Here's how the part is built. I have some questions about the finished solid (model axes, mm). Round coordinates to 2 decimals unless told otherwise and drop trailing zeros. Loops run counter-clockwise (first coordinate to the right, second up) from the corner with the lowest first, then second, coordinate; pieces in that order, holes last. Notation, with made-up numbers: M 67,-38.75 L 103,-38.75 A20 ccw 103,-31.75 Z; hole C 16,7.25 d9. An arc over 180 degrees is marked long. Use a Markdown table: item, result.
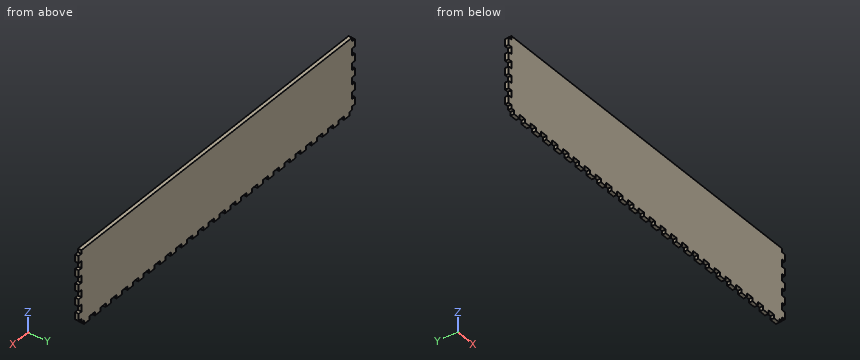
```python
from build123d import *

# Parameters (mm, degrees)
SKETCH001_W             = 500
SKETCH001_H             = 100
PAD001_DEPTH            = 5
SKETCH022_W             = 10
SKETCH022_H             = 5
PAD020_DEPTH            = 5
LINEARPATTERN002_COUNT  = 25
LINEARPATTERN002_PITCH  = 20
SKETCH023_W             = 10
SKETCH023_H             = 5
PAD021_DEPTH            = 5
LINEARPATTERN003_COUNT  = 5
LINEARPATTERN003_PITCH  = 20
SKETCH024_W             = 10
SKETCH024_H             = 5
PAD022_DEPTH            = 5
LINEARPATTERN004_COUNT  = 5
LINEARPATTERN004_PITCH  = 20
BODY001_PLACEMENT_ANGLE = 90


with BuildPart() as part:
    # Sketch001 → Pad001 (new body)
    with BuildSketch(Plane.XY):
        Rectangle(SKETCH001_W, SKETCH001_H)
    extrude(amount=PAD001_DEPTH)

    # Sketch022 (on DatumPlane) → Pad020 (join)
    with BuildSketch(Plane.XZ.offset(50)):
        with Locations((-240, 2.5)):
            Rectangle(SKETCH022_W, SKETCH022_H)
    pad020 = extrude(amount=PAD020_DEPTH)

    # LinearPattern002: Pad020 ×25
    with Locations(*[(i * LINEARPATTERN002_PITCH, 0, 0) for i in range(1, LINEARPATTERN002_COUNT)]):
        add(pad020)

    # Sketch023 (on DatumPlane) → Pad021 (join)
    with BuildSketch(Plane.YZ.offset(250)):
        with Locations((-40, 2.5)):
            Rectangle(SKETCH023_W, SKETCH023_H)
    pad021 = extrude(amount=PAD021_DEPTH)

    # LinearPattern003: Pad021 ×5
    with Locations(*[(0, i * LINEARPATTERN003_PITCH, 0) for i in range(1, LINEARPATTERN003_COUNT)]):
        add(pad021)

    # Sketch024 (on DatumPlane) → Pad022 (join)
    with BuildSketch(Plane(origin=(-250, 0, 0), x_dir=(0, -1, 0), z_dir=(-1, 0, 0))):
        with Locations((-40, 2.5)):
            Rectangle(SKETCH024_W, SKETCH024_H)
    pad022 = extrude(amount=PAD022_DEPTH)

    # LinearPattern004: Pad022 ×5
    with Locations(*[(0, -i * LINEARPATTERN004_PITCH, 0) for i in range(1, LINEARPATTERN004_COUNT)]):
        add(pad022)


with BuildPart() as part_1:
    # Body001 placement: moved
    add(part.part.moved(Location((0, 150, 55))).rotate(Axis((0, 150, 55), (1, 0, 0)), BODY001_PLACEMENT_ANGLE))


solid = part_1.part
```
Q1. Will these pins go through, and if not, where does the flat tip stop? P1, Ø2.5, axis at x = 210.5, y = 148, coming from the -Z side; P2, Ø2.5, axis at y = 146.5, z = 3.5, coming from the -X side; P3, Ø2.5, axis at y = 147.5, z = 7.5, coming from the -X side.
Return value:
| item | result |
|---|---|
| P1 | stops at z = 5 |
| P2 | stops at x = -245 |
| P3 | stops at x = -250 |
Q2. Imagine slicing it at A-A, the plane z = 65.5. Please give me the cut outline in (x, y).
Return value:
| item | result |
|---|---|
| outline | M -250,145 L 250,145 L 250,150 L -250,150 Z |
Q3. I need wall thicknesses on line 1 (X direction, y = 146.5, z = 48.5); line 2 (Z direction, x = 153, y = 145.35). Which ranges of each line are inside material? Lowest first, please. Write a range as from..to.
Return value:
| item | result |
|---|---|
| line 1 | x = -250..250 |
| line 2 | z = 5..105 |
Q4. Imagine slicing it at B-B, the plane x = 90. Please give me the cut outline in (y, z).
Return value:
| item | result |
|---|---|
| outline | M 145,5 L 150,5 L 150,105 L 145,105 Z |
